Geometry: final body of the model. Coordinates: model frame, mm. Coordinates: 2 decimals unless noted, no trailing zeros. Order: outer loops, then holes, each group sorted by start corner. A loop starts at its lowest first (then second) coordinate and runs counter-clockwise, first axis right, second up. Notation, with made-up numbers: (57.5, 21) -> (85.5, 21) arc R7 cw to (85.5, 26) -> close; hole circle Ø10 at (53, 35). An arc over 180 degrees is marked (long way). Answer in a Markdown table with one row per item. Add a question column.
1) Section query B-B on z = -53.5. Return the cut outline in (x, y), then the cut area to 3 significant figures.
2) Contact query for flat-ended pins moving along their axis: P1, Ø4, axis at y = 3, z = -130.5, coming from the -X side; P2, Ø5, axis at x = -1, z = -7, coming from the -Y side; P3, Ø1.5, axis at x = 2.5, z = -54.5, coming from the +Y side; P4, Ø5.5, axis at y = 1.5, z = 0, coming from the +X side. Output: stop coordinate, or through.
3) Section query A-A on z = -129. Return the cut outline in (x, y), then the cut area to 3 significant figures.
4) Ray query, line 1 (X direction, y = -1, z = -23); line 2 (Y direction, x = 3, z = -26); line 3 (Y direction, x = 2.75, z = -8). Return the intervals inside material, ascending. Write a range as from..to.
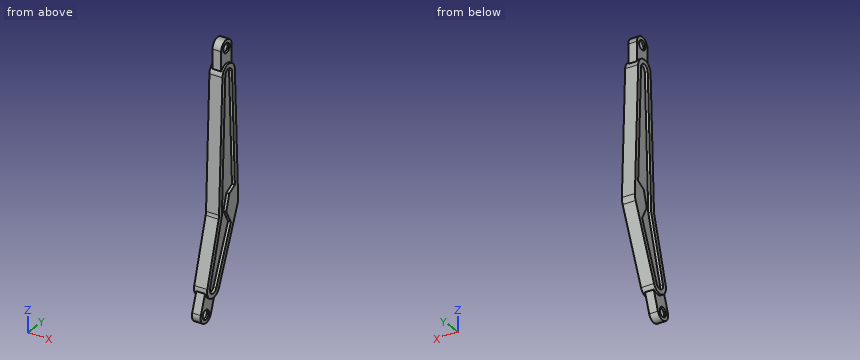
```python
from build123d import *
from build123d.topology import SkipClean

# Parameters (mm, degrees)
SKETCH1_R           = 3.25
BOSS_EXTRUDE1_DEPTH = 3
BOSS_EXTRUDE2_START = -4.5
BOSS_EXTRUDE2_DEPTH = 9
CUT_EXTRUDE1_DEPTH  = 2
FILLET1_R           = 10
CUT_EXTRUDE2_DEPTH  = 17
CHAMFER1_SIZE       = 1.5
CHAMFER1_SIZE_2     = 1.435934089
CUT_EXTRUDE3_DEPTH  = 17
CHAMFER2_SIZE       = 1.435934089


with BuildPart() as part:
    # Sketch1 → Boss-Extrude1 (new, symmetric)
    with BuildSketch(Plane(origin=(0, 0, 0), x_dir=(0, 0, -1), z_dir=(1, 0, 0))):
        with BuildLine():
            Line((105, 10), (16.24350989, 6.494937476))
            ThreePointArc((16.24350989, 6.494937476), (14.574337558, 6.208206195), (13.035898385, 5.5))
            Line((13.035898385, 5.5), (0, 5.5))
            ThreePointArc((0, 5.5), (-5.5, 0), (0, -5.5))
            Line((0, -5.5), (13.035898385, -5.5))
            ThreePointArc((13.035898385, -5.5), (14.574337558, -6.208206195), (16.24350989, -6.494937476))
            Line((16.24350989, -6.494937476), (106.559228351, -10.061575135))
            Line((106.559228351, -10.061575135), (148.580824133, -22.31516659))
            ThreePointArc((148.580824133, -22.31516659), (150.199105044, -22.57193923), (151.830180598, -22.41586927))
            Line((151.830180598, -22.41586927), (164.118536879, -26.766840037))
            ThreePointArc((164.118536879, -26.766840037), (171.138866131, -23.417963033), (167.789989128, -16.397633781))
            Line((167.789989128, -16.397633781), (155.501632847, -12.046663013))
            ThreePointArc((155.501632847, -12.046663013), (154.332173391, -10.899000225), (152.912873821, -10.08024872))
            Line((152.912873821, -10.08024872), (105, 10))
        make_face()
        Circle(SKETCH1_R, mode=Mode.SUBTRACT)
        with Locations((165.954263003, -21.582236909)):
            Circle(SKETCH1_R, mode=Mode.SUBTRACT)
    extrude(amount=BOSS_EXTRUDE1_DEPTH, both=True)

    # Boss-Extrude2: read off the stored shape, not the designer's step
    # Boss-Extrude2 outline → Boss-Extrude2 (add)
    with SkipClean():  # the faces are left unmerged after this step: merging them gives an invalid solid
        with BuildSketch(Plane(origin=(0, 0, 0), x_dir=(0, 0, -1), z_dir=(1, 0, 0)).offset(BOSS_EXTRUDE2_START)):
            with BuildLine():
                ThreePointArc((148.580824133, -22.31516659), (156.527711861, -18.244553046), (152.912873821, -10.08024872))
                Line((152.912873821, -10.08024872), (105, 10))
                Line((105, 10), (16.24350989, 6.494937476))
                ThreePointArc((16.24350989, 6.494937476), (10, 0), (16.24350989, -6.494937476))
                Line((16.24350989, -6.494937476), (106.559228351, -10.061575135))
                Line((106.559228351, -10.061575135), (148.580824133, -22.31516659))
            make_face()
        extrude(amount=BOSS_EXTRUDE2_DEPTH)

    # Sketch2 → Cut-Extrude1 (cut)
    with SkipClean():  # the faces are left unmerged after this step: merging them gives an invalid solid
        with BuildSketch(Plane(origin=(4.5, 0, 0), x_dir=(0, 0, -1), z_dir=(1, 0, 0))):
            with BuildLine():
                Line((95.980965998, 0.663794286), (92.809228462, 6.516238621))
                Line((92.809228462, 6.516238621), (16.361889941, 3.497274026))
                ThreePointArc((16.361889941, 3.497274026), (13, 0), (16.361889941, -3.497274026))
                Line((16.361889941, -3.497274026), (107.045551003, -7.078442023))
                Line((107.045551003, -7.078442023), (149.420653126, -19.435116719))
                ThreePointArc((149.420653126, -19.435116719), (153.699746519, -17.243247888), (151.753295266, -12.847084019))
                Line((151.753295266, -12.847084019), (115.449531272, 2.367795664))
                Line((115.449531272, 2.367795664), (106.52555447, -2.46856169))
                Line((106.52555447, -2.46856169), (95.980965998, 0.663794286))
            make_face()
        cut_extrude1 = extrude(amount=-CUT_EXTRUDE1_DEPTH, mode=Mode.SUBTRACT)

    # Mirror1: Cut-Extrude1 across plane
    with SkipClean():  # the faces are left unmerged after this step: merging them gives an invalid solid
        add(cut_extrude1.mirror(Plane(origin=(0, 0, 0), x_dir=(0, 0, 1), z_dir=(1, 0, 0))), mode=Mode.SUBTRACT)

    # Fillet1
    fillet1_edges = [part.edges().sort_by_distance(p)[0] for p in [
        (0, -10.061575135, -106.559228351),
        (0, 10, -105),
    ]]
    fillet(fillet1_edges, radius=FILLET1_R)

    # Sketch3 → Revolve1 (revolve)
    with SkipClean():  # the faces are left unmerged after this step: merging them gives an invalid solid
        with BuildSketch(Plane(origin=(0, 0, 0), x_dir=(0, 0, -1), z_dir=(1, 0, 0))):
            with BuildLine():
                ThreePointArc((4.5, 0), (0, 4.5), (-4.5, 0))
                Line((-4.5, 0), (-3.5, 0))
                ThreePointArc((-3.5, 0), (0, 3.5), (3.5, 0))
                Line((3.5, 0), (4.5, 0))
            make_face()
        revolve(axis=Axis((0, 0, 4.5), (0, 0, -1)))

    # Sketch4 → Cut-Extrude2 (cut)
    with SkipClean():  # the faces are left unmerged after this step: merging them gives an invalid solid
        with BuildSketch(Plane(origin=(0, 5.5, 0), x_dir=(1, 0, 0), z_dir=(0, 1, 0))):
            Polygon((3, 0), (3, -6.291238928), (6.747077204, -6.291238928), (6.747077204, 6.985365783), (3, 6.985365783), align=None)
            Polygon((-5.881309599, 6.985365783), (-5.881309599, -6.291238928), (-3, -6.291238928), (-3, 0), (-3, 6.985365783), align=None)
        extrude(amount=-CUT_EXTRUDE2_DEPTH, mode=Mode.SUBTRACT)

    # Chamfer1
    # the kernel refuses this chamfer: 1.5, 1.435934089 mm, written as the material it takes off along each edge
    with BuildSketch(Plane(origin=(3, 0, 0), x_dir=(0, 0, -1), z_dir=(0, 1, 0))) as chamfer1_piece_1:
        with BuildLine():
            Line((1.802775638 + CHAMFER1_SIZE, 0), (2.915614393, 1.063716779))
            ThreePointArc((2.915614393, 1.063716779), (2.427398497, 0.478544758), (1.802775638, 0))
            Line((1.802775638, 0), (1.802775638 + CHAMFER1_SIZE, 0))
        make_face()
    revolve(axis=Axis((3, 0, 0), (-1, 0, 0)), mode=Mode.SUBTRACT)
    with BuildSketch(Plane(origin=(-3, 0, 0), x_dir=(0, 0, 1), z_dir=(0, 1, 0))) as chamfer1_piece_2:
        with BuildLine():
            Line((1.802775638 + CHAMFER1_SIZE_2, 0), (3.00448024, 1.204701004))
            ThreePointArc((3.00448024, 1.204701004), (2.490248254, 0.540596895), (1.802775638, 0))
            Line((1.802775638, 0), (1.802775638 + CHAMFER1_SIZE_2, 0))
        make_face()
    revolve(axis=Axis((-3, 0, 0), (1, 0, 0)), mode=Mode.SUBTRACT)

    # Sketch5 → Revolve2 (revolve)
    with SkipClean():  # the faces are left unmerged after this step: merging them gives an invalid solid
        with BuildSketch(Plane(origin=(0, 0, 0), x_dir=(0, 0, -1), z_dir=(1, 0, 0))):
            with BuildLine():
                Line((169.454263003, -21.582236909), (170.454263003, -21.582236909))
                ThreePointArc((170.454263003, -21.582236909), (165.954263003, -17.082236909), (161.454263003, -21.582236909))
                Line((161.454263003, -21.582236909), (162.454263003, -21.582236909))
                ThreePointArc((162.454263003, -21.582236909), (165.954263003, -18.082236909), (169.454263003, -21.582236909))
            make_face()
        revolve(axis=Axis((0, -21.582236909, -170.454263003), (0, 0, 1)))

    # Sketch6 → Cut-Extrude3 (cut)
    with SkipClean():  # the faces are left unmerged after this step: merging them gives an invalid solid
        with BuildSketch(Plane(origin=(0, 38.220593136, -13.532866369), x_dir=(1, 0, 0), z_dir=(0, 0.9426551142039149, -0.33376838625790206))):
            Polygon((-6.767171252, 154.311979975), (-3, 154.311979975), (-3, 163.641103129), (-3, 169.141103129), (3, 169.141103129), (3, 154.311979975), (6.783794008, 154.311979975), (6.783794008, 170.859793321), (-6.767171252, 170.859793321), align=None)
        extrude(amount=-CUT_EXTRUDE3_DEPTH, mode=Mode.SUBTRACT)

    # Chamfer2
    # the kernel refuses this chamfer: 1.5, 1.435934089 mm, written as the material it takes off along each edge
    with BuildSketch(Plane(origin=(3, -21.582236909, -165.954263003), x_dir=(0, 0, -1), z_dir=(0, 1, 0))) as chamfer2_piece_1:
        with BuildLine():
            Line((1.802775638 + CHAMFER2_SIZE, 0), (3.00448024, 1.204701004))
            ThreePointArc((3.00448024, 1.204701004), (2.490248254, 0.540596895), (1.802775638, 0))
            Line((1.802775638, 0), (1.802775638 + CHAMFER2_SIZE, 0))
        make_face()
    revolve(axis=Axis((3, -21.582236909, -165.954263003), (-1, 0, 0)), mode=Mode.SUBTRACT)
    with BuildSketch(Plane(origin=(-3, -21.582236909, -165.954263003), x_dir=(0, 0, 1), z_dir=(0, 1, 0))) as chamfer2_piece_2:
        with BuildLine():
            Line((1.802775638 + CHAMFER2_SIZE, 0), (3.00448024, 1.204701004))
            ThreePointArc((3.00448024, 1.204701004), (2.490248254, 0.540596895), (1.802775638, 0))
            Line((1.802775638, 0), (1.802775638 + CHAMFER2_SIZE, 0))
        make_face()
    revolve(axis=Axis((-3, -21.582236909, -165.954263003), (1, 0, 0)), mode=Mode.SUBTRACT)

    # Sketch5<6> → Cut-Revolve1 (revolve, cut)
    with SkipClean():  # the faces are left unmerged after this step: merging them gives an invalid solid
        with BuildSketch(Plane(origin=(0, 0, 0), x_dir=(0, 0, -1), z_dir=(1, 0, 0))):
            with BuildLine():
                Line((162.454263003, -21.582236909), (169.454263003, -21.582236909))
                ThreePointArc((169.454263003, -21.582236909), (165.954263003, -18.082236909), (162.454263003, -21.582236909))
            make_face()
        revolve(axis=Axis((0, -21.582236909, -170.454263003), (0, 0, 1)), mode=Mode.SUBTRACT)

    # Sketch3<6> → Cut-Revolve2 (revolve, cut)
    with SkipClean():  # the faces are left unmerged after this step: merging them gives an invalid solid
        with BuildSketch(Plane(origin=(0, 0, 0), x_dir=(0, 0, -1), z_dir=(1, 0, 0))):
            with BuildLine():
                ThreePointArc((3.5, 0), (0, 3.5), (-3.5, 0))
                Line((-3.5, 0), (3.5, 0))
            make_face()
        revolve(axis=Axis((0, 0, 4.5), (0, 0, -1)), mode=Mode.SUBTRACT)


solid = part.part
```
Result:
| question | item | result |
|---|---|---|
| 1 | outline | (-4.5, -7.97) -> (4.5, -7.97) -> (4.5, -4.96) -> (2.5, -4.96) -> (2.5, 4.96) -> (4.5, 4.96) -> (4.5, 7.97) -> (-4.5, 7.97) -> (-4.5, 4.96) -> (-2.5, 4.96) -> (-2.5, -4.96) -> (-4.5, -4.96) -> close |
| 1 | area | 104 mm2 |
| 2 | P1 | through |
| 2 | P2 | y = -5.5 |
| 2 | P3 | y = 8.04 |
| 2 | P4 | x = 3 |
| 3 | outline | (-4.5, -16.61) -> (4.5, -16.61) -> (4.5, -13.48) -> (2.5, -13.48) -> (2.5, -3.31) -> (4.5, -3.31) -> (4.5, -0.06) -> (-4.5, -0.06) -> (-4.5, -3.31) -> (-2.5, -3.31) -> (-2.5, -13.48) -> (-4.5, -13.48) -> close |
| 3 | area | 108 mm2 |
| 4 | line 1 | -2.5..2.5 |
| 4 | line 2 | -6.88..-3.88, 3.88..6.88 |
| 4 | line 3 | -5.5..5.5 |
